Could you check a few things on this model? Use its own coordinates, in mm. A direction names the side the tool comes from. Round coordinates to 2 decimals unless told otherwise and drop trailing zeros. Loops run counter-clockwise (first coordinate to the right, second up) from the corner with the lowest first, then second, coordinate; pieces in that order, holes last. Notation, with made-up numbers: M 57.5,41 L 116.5,41 A34 ccw 116.5,78 Z; hole C 0,-23 d8. An arc over 180 degrees is marked long. Answer in a Markdown table with one row per item.
Autodesk Inventor part; units mm, degrees
ref_plane "Start Plane" through (0, 0, 34.94) normal (0, 0, 1) x (1, 0, 0)
ref_plane "End Plane" through (0, 0, 464.94) normal (0, 0, 1) x (1, 0, 0)
ref_plane "Work Plane4" through (1040, 29, 34.94) normal (0, 0, -1) x (-1, 0, 0)
ref_plane "Start Plane" through (0, 0, 34.94) normal (0, 0, 1) x (1, 0, 0)
ref_plane "End Plane" through (0, 0, 464.94) normal (0, 0, 1) x (1, 0, 0)
sketch "Sketch" plane through (0, 0, 0) normal (0, 0, 1) x (1, 0, 0)
  line L0 (-25, -21) -> (-25, 21)
  line L1 (-21, 25) -> (21, 25)
  line L2 (25, 21) -> (25, -21)
  line L3 (21, -25) -> (-21, -25)
  arc A0 (-25, -21) -> (-21, -25) centre (-21, -21) ccw
  arc A1 (25, 21) -> (21, 25) centre (21, 21) ccw
  arc A2 (-21, 25) -> (-25, 21) centre (-21, 21) ccw
  arc A3 (21, -25) -> (25, -21) centre (21, -21) ccw
  arc A4 (-21, 23) -> (-23, 21) centre (-21, 21) ccw
  line L4 (-21, 23) -> (21, 23)
  arc A5 (23, 21) -> (21, 23) centre (21, 21) ccw
  line L5 (23, 21) -> (23, -21)
  arc A6 (21, -23) -> (23, -21) centre (21, -21) ccw
  line L6 (21, -23) -> (-21, -23)
  arc A7 (-23, -21) -> (-21, -23) centre (-21, -21) ccw
  line L7 (-23, -21) -> (-23, 21)
  line L8 (0, 36.1598) -> (0, -36.1598) construction
  line L9 (-36.1598, 0) -> (36.1598, 0) construction
  dimension "d7" = 4
  dimension "d9" = 50
  dimension "d11" = 50
  dimension "d12" = 2
  dimension "d15" = 25
  dimension "d16" = 25
extrude "Body" add sketch "Sketch" along normal up to surface (430 mm away) from surface at 34.94
sketch "Sketch3" plane through (0, 0, 0) normal (0, 0, 1) x (1, 0, 0)
  line L0 (0, 0) -> (10, 0)
ref_plane "Work Plane3" through (0, 0, 0) normal (0, -1, 0) x (1, 0, 0)
sketch "Sketch4" plane through (0, 0, 0) normal (0, -1, 0) x (1, 0, 0)
  line L0 (-2, 34.94) -> (12, 34.94)
  line L1 (-2, 464.94) -> (12, 464.94)
  dimension "d18" = 430
ref_plane "Work Plane4" through (1040, 29, 34.94) normal (0, 0, -1) x (-1, 0, 0)
split "Split1" plane through (1040, 29, 34.94) removes the side toward (0, 0, -1)
ref_plane "Work Plane5" through (-1270, 29, 464.94) normal (0, 0, 1) x (1, 0, 0)
split "Split2" plane through (-1270, 29, 464.94) removes the side toward (0, 0, 1)
ref_plane "Work Plane9" through (-114.5, -25, 249.94) normal (0, 1, 0) x (0, 0, -1)
sketch "Sketch5" plane through (-114.5, -25, 249.94) normal (0, 1, 0) x (0, 0, -1)
  circle A0 centre (40, -115) radius 6
  circle A1 centre (-40, -115) radius 6
  point P0 (249.94, -114.5)
extrude "Extrusion2" cut sketch "Sketch5" along normal through all
equation "\"d7\" = G_IR"
equation "\"d9\" = G_W"
equation "\"d11\" = G_H"
equation "\"d12\" = G_T"
equation "\"d15\" = 0.5 * d9"
equation "\"d16\" = 0.5 * d11"
equation "\"d3\" = G_L"
equation "\"G_W\" = 50"
equation "\"G_H\" = 50"
equation "\"G_T\" = 2"
equation "\"G_IR\" = 4"
equation "\"G_L\" = d18"
equation "\"G_OFFSET_START\" = -34.94003"
equation "\"G_OFFSET_END\" = -35.05997"
equation "\"d13\" = -G_OFFSET_START"
equation "\"d14\" = G_OFFSET_END + B_L"
properties part number "ISO 10799-2 - 50x50x2 - 430" material "Steel, Galvanized"
1) Which directions (+Z, -Z, +X, -X, +Y, -Y) give clear straight access to the entire face, cutting with the end or side of a thin tool? Please do faces 4 (the face through (0, 25, 247)), 5 (the face through (0, -23, 247)).
Computed:
| item | result |
|---|---|
| face 4 | +Z, -Z, +X, -X, +Y |
| face 5 | +Z, -Z |
2) I want a section at A-A, the plane y = 4.5. Please give me the cut outline in (x, z), plus the area to 3 significant figures.
Computed:
| item | result |
|---|---|
| outline | M -25,34.94 L -23,34.94 L -23,464.94 L -25,464.94 Z; M 23,34.94 L 25,34.94 L 25,464.94 L 23,464.94 Z |
| area | 1,720 mm² |
3) I need wall thicknesses on line 1 (X direction, y = 10, z = 385.5); line 2 (Z direction, x = 0.5, y = -23.75). Which ranges of each line are inside material? Lowest first, please.
Computed:
| item | result |
|---|---|
| line 1 | x = -25 to -23, 23 to 25 |
| line 2 | z = 34.94 to 203.94, 215.94 to 283.94, 295.94 to 464.94 |
4) Will this pin go through, and if not, where does the flat tip stop? P1, Ø14, axis at x = 0.5, z = 289.94, coming from the -Y side.
Computed:
| item | result |
|---|---|
| P1 | stops at y = -25 |
5) If we mould it in two halves opening along X, with no side actions, what happens to faces 1 (the face through (-25, 0, 247)), 2 (the face through (-23, 0, 247)), 3 (the face through (0, 24, 464.94))? For each: released by +X, released by -X, zero draft, split by the parting line, or undercut.
Computed:
| item | result |
|---|---|
| face 1 | released by -X |
| face 2 | undercut |
| face 3 | zero draft |
6) I want a section at C-C, the plane z = 342.5. Please give me the cut outline in (x, y).
Computed:
| item | result |
|---|---|
| outline | M -25,-21 A4 ccw -21,-25 L 21,-25 A4 ccw 25,-21 L 25,21 A4 ccw 21,25 L -21,25 A4 ccw -25,21 Z; hole M -23,-21 A2 ccw -21,-23 L 21,-23 A2 ccw 23,-21 L 23,21 A2 ccw 21,23 L -21,23 A2 ccw -23,21 Z |
7) I want a section at D-D, the plane z = 209.94. Please give me the cut outline in (x, y).
Computed:
| item | result |
|---|---|
| outline | M -25,-21 A4 ccw -21,-25 L -5.5,-25 L -5.5,-23 L -21,-23 A2 cw -23,-21 L -23,21 A2 cw -21,23 L -5.5,23 L -5.5,25 L -21,25 A4 ccw -25,21 Z; M 6.5,-25 L 21,-25 A4 ccw 25,-21 L 25,21 A4 ccw 21,25 L 6.5,25 L 6.5,23 L 21,23 A2 cw 23,21 L 23,-21 A2 cw 21,-23 L 6.5,-23 Z |
